from build123d import *

# Parameters (mm, degrees)
F0_R          = 31
F1_DEPTH      = 2
F2_R          = 22
F3_DEPTH      = 91
F4_W          = 67.803
F4_H          = 21
F5_DEPTH      = 25
F7_DEPTH      = 20.501
F7_DEPTH_BACK = 43.7
F8_R          = 17
F9_DEPTH      = 63
F10_R         = 31
F11_DEPTH     = 2


with BuildPart() as f1:
    # F0 (on Top) → F1 (new body)
    with BuildSketch(Plane.XY):
        Circle(F0_R)
    extrude(amount=F1_DEPTH)

    # F2 (on face) → F3 (join)
    with BuildSketch(Plane.XY.offset(2)):
        Circle(F2_R)
    extrude(amount=F3_DEPTH)

    # F4 (on face) → F5 (cut)
    with BuildSketch(Plane.XY.offset(93)):
        Rectangle(F4_W, F4_H)
    extrude(amount=-F5_DEPTH, mode=Mode.SUBTRACT)

    # F6 (on face) → F7 (cut, two sides)
    with BuildSketch(Plane.XZ.offset(-10.5)) as f7_sk:
        with BuildLine():
            ThreePointArc((0, 80), (-2, 78), (0, 76))
            Line((0, 76), (0, 78))
            Line((0, 78), (0, 80))
        make_face()
        with BuildLine():
            Line((0, 78), (0, 76))
            ThreePointArc((0, 76), (1.4142135624, 76.5857864376), (2, 78))
            ThreePointArc((2, 78), (1.4142135624, 79.4142135624), (0, 80))
            Line((0, 80), (0, 78))
        make_face()
    extrude(amount=-F7_DEPTH, mode=Mode.SUBTRACT)
    extrude(f7_sk.sketch, amount=F7_DEPTH_BACK, mode=Mode.SUBTRACT)

    # F8 (on face) → F9 (cut)
    with BuildSketch(Plane(origin=(0, 0, 0), x_dir=(1, 0, 0), z_dir=(0, 0, -1))):
        Circle(F8_R)
    extrude(amount=-F9_DEPTH, mode=Mode.SUBTRACT)

    # F10 (on face) → F11 (join)
    with BuildSketch(Plane(origin=(0, 0, 0), x_dir=(1, 0, 0), z_dir=(0, 0, -1))):
        Circle(F10_R)
    extrude(amount=-F11_DEPTH)


solid = f1.part
Source: CAD feature listing. Evaluate the final solid. Frame: model axes, mm. A direction names the side the tool comes from. Give positions to 0.01 mm unless a question says otherwise; leave off trailing zeros. Order: outer loops, then holes, each group sorted by start corner. A loop starts at its lowest first (then second) coordinate and runs counter-clockwise, first axis right, second up. Notation, with made-up numbers: (-34, 48) -> (3, 48) arc R10 ccw to (3, 54) -> close; hole circle Ø7 at (77, -7). An arc over 180 degrees is marked (long way). Use a Markdown table: item, result.
1) Section query A-A, the plane y = 0. Return the cut outline in (x, z).
Answer list:
| item | result |
|---|---|
| outline | (-31, 0) -> (31, 0) -> (31, 2) -> (22, 2) -> (22, 68) -> (-22, 68) -> (-22, 2) -> (-31, 2) -> close; hole (-17, 2) -> (17, 2) -> (17, 63) -> (-17, 63) -> close |
2) Section query B-B, the plane x = -8.5. Return the cut outline in (y, z).
Answer list:
| item | result |
|---|---|
| outline | (-29.81, 0) -> (29.81, 0) -> (29.81, 2) -> (20.29, 2) -> (20.29, 93) -> (10.5, 93) -> (10.5, 68) -> (-10.5, 68) -> (-10.5, 93) -> (-20.29, 93) -> (-20.29, 2) -> (-29.81, 2) -> close; hole (-14.72, 2) -> (14.72, 2) -> (14.72, 63) -> (-14.72, 63) -> close |
3) Reachability of faces 1 (the flat face through (0, 10.5, 81)), 2 (the cylindrical face through (-21.98, 0.97, 46.86)), 3 (the cylindrical face through (9.139, -14.334, 32.073)) from +Z, -Z, +X, -X, +Y, -Y: full face, straight path, thin tool, end or side. Return the list, or none.
Answer list:
| item | result |
|---|---|
| face 1 | +Z, +X, -X |
| face 2 | +Z |
| face 3 | none |
4) Mould query, pull axis Y, two halves, no side actions, for faces 4 (the cylindrical face through (-4.036, 30.736, 0.986)), 5 (the flat face through (0, 0, 63)), 6 (the flat face through (-21.1, 7.3, 2)). Classes: +Y half, -Y half, draft (parallel to the pull), parting line (faces both ways), or undercut.
Answer list:
| item | result |
|---|---|
| face 4 | parting line |
| face 5 | undercut |
| face 6 | draft |
5) Section query C-C, the plane z = 17. Return the cut outline in (x, y), then the cut area to 3 significant figures.
Answer list:
| item | result |
|---|---|
| outline | circle Ø44 at (0, 0); hole circle Ø34 at (0, 0) |
| area | 613 mm² |
6) Ray query, line 1 along Z through (x, y) = (-12, 6); line 2 along Y through (x, z) = (0, 19); line 3 along Z through (x, y) = (10, -13.5). Return the intervals inside material, ascending. Write a range as [from, to].
Answer list:
| item | result |
|---|---|
| line 1 | [0, 2], [63, 68] |
| line 2 | [-22, -17], [17, 22] |
| line 3 | [0, 2], [63, 93] |
7) Contact query for flat-ended pins moving along their axis: P1, Ø3, axis at y = -14, z = 37, coming from the -X side; P2, Ø5, axis at x = 9, y = 4.5, coming from the +Z side; P3, Ø20, axis at x = 5.5, z = 80, coming from the +Y side; P4, Ø1.5, axis at x = 23, y = 24, coming from the +Z side. Output: stop coordinate, or through.
Answer list:
| item | result |
|---|---|
| P1 | x = -18.1 |
| P2 | z = 68 |
| P3 | y = 22 |
| P4 | through |
8) Section query D-D, the plane y = -14. Return the cut outline in (x, z).
Answer list:
| item | result |
|---|---|
| outline | (-27.66, 0) -> (27.66, 0) -> (27.66, 2) -> (16.97, 2) -> (16.97, 93) -> (-16.97, 93) -> (-16.97, 2) -> (-27.66, 2) -> close; hole (-9.64, 2) -> (9.64, 2) -> (9.64, 63) -> (-9.64, 63) -> close; hole circle Ø4 at (0, 78) |
